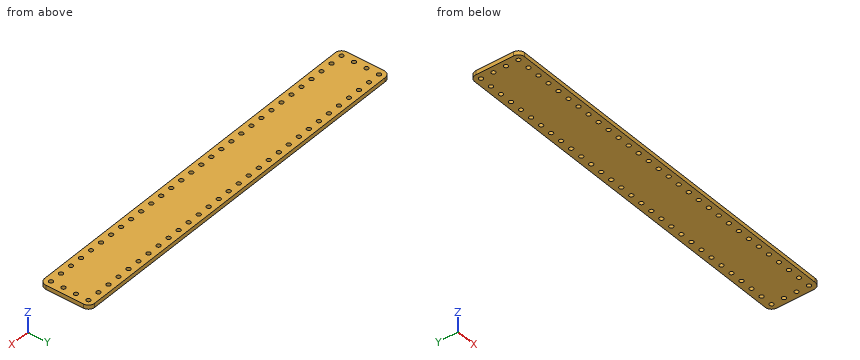
from build123d import *

# Parameters (mm, degrees)
MODEL_R                 = 1.5
SALIENTE_EXTRUIR1_DEPTH = 3


with BuildPart() as part:
    # Model → Saliente-Extruir1 (new body)
    with BuildSketch(Plane.XY):
        with BuildLine():
            Line((-105.943383637, 101.056539338), (-105.943383637, 74.056539338))
            ThreePointArc((-105.943383637, 74.056539338), (-104.625364152, 70.874558823), (-101.443383637, 69.556539338))
            Line((-101.443383637, 69.556539338), (159.556616363, 69.556539338))
            ThreePointArc((159.556616363, 69.556539338), (162.738596878, 70.874558823), (164.056616363, 74.056539338))
            Line((164.056616363, 74.056539338), (164.056616363, 101.056539338))
            ThreePointArc((164.056616363, 101.056539338), (162.738596878, 104.238519853), (159.556616363, 105.556539338))
            Line((159.556616363, 105.556539338), (-101.443383637, 105.556539338))
            ThreePointArc((-101.443383637, 105.556539338), (-104.625364152, 104.238519853), (-105.943383637, 101.056539338))
        make_face()
        with Locations((-101.443383637, 101.056539338)):
            Circle(MODEL_R, mode=Mode.SUBTRACT)
        with Locations((-92.443383637, 101.056539338)):
            Circle(MODEL_R, mode=Mode.SUBTRACT)
        with Locations((-83.443383637, 101.056539338)):
            Circle(MODEL_R, mode=Mode.SUBTRACT)
        with Locations((-74.443383637, 101.056539338)):
            Circle(MODEL_R, mode=Mode.SUBTRACT)
        with Locations((-65.443383637, 101.056539338)):
            Circle(MODEL_R, mode=Mode.SUBTRACT)
        with Locations((-56.443383637, 101.056539338)):
            Circle(MODEL_R, mode=Mode.SUBTRACT)
        with Locations((-47.443383637, 101.056539338)):
            Circle(MODEL_R, mode=Mode.SUBTRACT)
        with Locations((-38.443383637, 101.056539338)):
            Circle(MODEL_R, mode=Mode.SUBTRACT)
        with Locations((-101.443383637, 92.056539338)):
            Circle(MODEL_R, mode=Mode.SUBTRACT)
        with Locations((-101.443383637, 83.056539338)):
            Circle(MODEL_R, mode=Mode.SUBTRACT)
        with Locations((-101.443383637, 74.056539338)):
            Circle(MODEL_R, mode=Mode.SUBTRACT)
        with Locations((-92.443383637, 74.056539338)):
            Circle(MODEL_R, mode=Mode.SUBTRACT)
        with Locations((-83.443383637, 74.056539338)):
            Circle(MODEL_R, mode=Mode.SUBTRACT)
        with Locations((-74.443383637, 74.056539338)):
            Circle(MODEL_R, mode=Mode.SUBTRACT)
        with Locations((-65.443383637, 74.056539338)):
            Circle(MODEL_R, mode=Mode.SUBTRACT)
        with Locations((-56.443383637, 74.056539338)):
            Circle(MODEL_R, mode=Mode.SUBTRACT)
        with Locations((-47.443383637, 74.056539338)):
            Circle(MODEL_R, mode=Mode.SUBTRACT)
        with Locations((-38.443383637, 74.056539338)):
            Circle(MODEL_R, mode=Mode.SUBTRACT)
        with Locations((-29.443383637, 101.056539338)):
            Circle(MODEL_R, mode=Mode.SUBTRACT)
        with Locations((-29.443383637, 74.056539338)):
            Circle(MODEL_R, mode=Mode.SUBTRACT)
        with Locations((-20.443383637, 101.056539338)):
            Circle(MODEL_R, mode=Mode.SUBTRACT)
        with Locations((-20.443383637, 74.056539338)):
            Circle(MODEL_R, mode=Mode.SUBTRACT)
        with Locations((-11.443383637, 101.056539338)):
            Circle(MODEL_R, mode=Mode.SUBTRACT)
        with Locations((-2.443383637, 101.056539338)):
            Circle(MODEL_R, mode=Mode.SUBTRACT)
        with Locations((6.556616363, 101.056539338)):
            Circle(MODEL_R, mode=Mode.SUBTRACT)
        with Locations((15.556616363, 101.056539338)):
            Circle(MODEL_R, mode=Mode.SUBTRACT)
        with Locations((24.556616363, 101.056539338)):
            Circle(MODEL_R, mode=Mode.SUBTRACT)
        with Locations((33.556616363, 101.056539338)):
            Circle(MODEL_R, mode=Mode.SUBTRACT)
        with Locations((42.556616363, 101.056539338)):
            Circle(MODEL_R, mode=Mode.SUBTRACT)
        with Locations((51.556616363, 101.056539338)):
            Circle(MODEL_R, mode=Mode.SUBTRACT)
        with Locations((-11.443383637, 74.056539338)):
            Circle(MODEL_R, mode=Mode.SUBTRACT)
        with Locations((-2.443383637, 74.056539338)):
            Circle(MODEL_R, mode=Mode.SUBTRACT)
        with Locations((6.556616363, 74.056539338)):
            Circle(MODEL_R, mode=Mode.SUBTRACT)
        with Locations((15.556616363, 74.056539338)):
            Circle(MODEL_R, mode=Mode.SUBTRACT)
        with Locations((24.556616363, 74.056539338)):
            Circle(MODEL_R, mode=Mode.SUBTRACT)
        with Locations((33.556616363, 74.056539338)):
            Circle(MODEL_R, mode=Mode.SUBTRACT)
        with Locations((42.556616363, 74.056539338)):
            Circle(MODEL_R, mode=Mode.SUBTRACT)
        with Locations((51.556616363, 74.056539338)):
            Circle(MODEL_R, mode=Mode.SUBTRACT)
        with Locations((60.556616363, 101.056539338)):
            Circle(MODEL_R, mode=Mode.SUBTRACT)
        with Locations((60.556616363, 74.056539338)):
            Circle(MODEL_R, mode=Mode.SUBTRACT)
        with Locations((69.556616363, 101.056539338)):
            Circle(MODEL_R, mode=Mode.SUBTRACT)
        with Locations((69.556616363, 74.056539338)):
            Circle(MODEL_R, mode=Mode.SUBTRACT)
        with Locations((78.556616363, 101.056539338)):
            Circle(MODEL_R, mode=Mode.SUBTRACT)
        with Locations((87.556616363, 101.056539338)):
            Circle(MODEL_R, mode=Mode.SUBTRACT)
        with Locations((96.556616363, 101.056539338)):
            Circle(MODEL_R, mode=Mode.SUBTRACT)
        with Locations((105.556616363, 101.056539338)):
            Circle(MODEL_R, mode=Mode.SUBTRACT)
        with Locations((114.556616363, 101.056539338)):
            Circle(MODEL_R, mode=Mode.SUBTRACT)
        with Locations((123.556616363, 101.056539338)):
            Circle(MODEL_R, mode=Mode.SUBTRACT)
        with Locations((132.556616363, 101.056539338)):
            Circle(MODEL_R, mode=Mode.SUBTRACT)
        with Locations((141.556616363, 101.056539338)):
            Circle(MODEL_R, mode=Mode.SUBTRACT)
        with Locations((78.556616363, 74.056539338)):
            Circle(MODEL_R, mode=Mode.SUBTRACT)
        with Locations((87.556616363, 74.056539338)):
            Circle(MODEL_R, mode=Mode.SUBTRACT)
        with Locations((96.556616363, 74.056539338)):
            Circle(MODEL_R, mode=Mode.SUBTRACT)
        with Locations((105.556616363, 74.056539338)):
            Circle(MODEL_R, mode=Mode.SUBTRACT)
        with Locations((114.556616363, 74.056539338)):
            Circle(MODEL_R, mode=Mode.SUBTRACT)
        with Locations((123.556616363, 74.056539338)):
            Circle(MODEL_R, mode=Mode.SUBTRACT)
        with Locations((132.556616363, 74.056539338)):
            Circle(MODEL_R, mode=Mode.SUBTRACT)
        with Locations((141.556616363, 74.056539338)):
            Circle(MODEL_R, mode=Mode.SUBTRACT)
        with Locations((150.556616363, 101.056539338)):
            Circle(MODEL_R, mode=Mode.SUBTRACT)
        with Locations((150.556616363, 74.056539338)):
            Circle(MODEL_R, mode=Mode.SUBTRACT)
        with Locations((159.556616363, 101.056539338)):
            Circle(MODEL_R, mode=Mode.SUBTRACT)
        with Locations((159.556616363, 92.056539338)):
            Circle(MODEL_R, mode=Mode.SUBTRACT)
        with Locations((159.556616363, 83.056539338)):
            Circle(MODEL_R, mode=Mode.SUBTRACT)
        with Locations((159.556616363, 74.056539338)):
            Circle(MODEL_R, mode=Mode.SUBTRACT)
    extrude(amount=SALIENTE_EXTRUIR1_DEPTH)


solid = part.part
CAD build for the part. Positions are in the model's coordinates, mm. Coordinates: 2 decimals unless noted, no trailing zeros. Answer as a JSON object with one key per item and string values. Group by question number.
1) Pin check, flat tips, straight feed: pin 1 Ø2.5 at (x, y) = (-74.44, 74.06) entering from -Z; pin 2 Ø3.5 at (x, y) = (105.56, 101.06) entering from -Z. Stop position of each tip, or through.
2) Wall check: line 1 (X direction, y = 92, z = 1.4); line 2 (Y direction, x = -75.5, z = 1.75); line 3 (Y direction, x = 7, z = 2.45). Give the ranges that are in metal, low to high. Write a range as from..to.
3) Saw through at A-A (z = 1.95). Give the number of separate pieces and of enclosed holes in the cut face, plus the area to 3 significant figures.
Values follow:
{
 "1": {"pin 1": "passes through", "pin 2": "stops at z = 0"},
 "2": {"line 1": "x = -105.94..-102.94, -99.94..158.06, 161.06..164.06", "line 2": "y = 69.56..72.99, 75.12..99.99, 102.12..105.56", "line 3": "y = 69.56..72.62, 75.49..99.62, 102.49..105.56"},
 "3": {"separate pieces": "1", "enclosed holes": "64", "area": "9,250 mm2"}
}
